```python
from build123d import *

# Parameters (mm, degrees)
EXTRUDE_1_DEPTH   = 2
HOLE_WIZARD_M61_D = 6.6
CHAMFER_1_SIZE    = 2


with BuildPart() as part:
    # Эскиз1 → Бобышка-Вытянуть1 (new body)
    with BuildSketch(Plane(origin=(0, 0, 0), x_dir=(1, 0, 0), z_dir=(0, 0, -1))):
        Polygon((0, 0), (0, 90), (90, 90), (90, 70), (20, 0), align=None)
    extrude(amount=EXTRUDE_1_DEPTH)

    # Отверстие с зазором M61 (through all)
    with Locations(Plane(origin=(0, 0, -2), x_dir=(1, 0, 0), z_dir=(0, 0, -1))):
        with Locations((40, 80), (10, 80), (10, 50), (10, 20), (70, 80), (40, 50)):
            Hole(HOLE_WIZARD_M61_D / 2)

    # Фаска1
    chamfer_1_edges = [part.edges().sort_by_distance(p)[0] for p in [
        (0, 0, -1),
        (0, -90, -1),
        (90, -90, -1),
    ]]
    chamfer(chamfer_1_edges, length=CHAMFER_1_SIZE)


solid = part.part
```
Input: part model. Units: mm. Frame: model coordinates. Coordinates: 2 decimals unless noted, no trailing zeros. Loops run counter-clockwise (first coordinate to the right, second up) from the corner with the lowest first, then second, coordinate; pieces in that order, holes last.
Q1. Mould query, pull axis Y, two halves, no side actions, for faces 1 (the flat face through (1, -1, -1)), 2 (the flat face through (36, -56, 0)), 3 (the cylindrical face through (12.619, -17.992, -0.986)), 4 (the flat face through (89, -89, -1)). Classes: +Y half, -Y half, draft (parallel to the pull), parting line (faces both ways), or undercut.
Results are:
face 1: +Y half
face 2: draft
face 3: undercut
face 4: -Y half
Q2. Line query: line 1 along Y through (x, z) = (10, -1.25); line 2 along X through (y, z) = (-80, -1.45); line 3 along Y through (x, z) = (38, -1.8). Output: solid intervals per line, ascending.
Results are:
line 1: y = -90 to -83.3, -76.7 to -53.3, -46.7 to -23.3, -16.7 to 0
line 2: x = 0 to 6.7, 13.3 to 36.7, 43.3 to 66.7, 73.3 to 90
line 3: y = -90 to -82.62, -77.38 to -52.62, -47.38 to -18
Q3. Section C-C, the plane z = -1.05. Return the cut outline in (x, y), and give its area (3 significant figures).
Results are:
outline: (0, -88) - (2, -90) - (88, -90) - (90, -88) - (90, -70) - (20, 0) - (2, 0) - (0, -2) - close; hole circle Ø6.6 at (10, -80); hole circle Ø6.6 at (10, -50); hole circle Ø6.6 at (10, -20); hole circle Ø6.6 at (40, -80); hole circle Ø6.6 at (40, -50); hole circle Ø6.6 at (70, -80)
area: 5,440 mm2
Q4. Section B-B, the plane y = -80. Return the cut outline in (x, z).
Results are:
outline: (0, -2) - (6.7, -2) - (6.7, 0) - (0, 0) - close; (13.3, -2) - (36.7, -2) - (36.7, 0) - (13.3, 0) - close; (43.3, -2) - (66.7, -2) - (66.7, 0) - (43.3, 0) - close; (73.3, -2) - (90, -2) - (90, 0) - (73.3, 0) - close
Q5. Section D-D, the plane x = 10. Return the cut outline in (y, z), and give its area (3 significant figures).
Results are:
outline: (-90, -2) - (-83.3, -2) - (-83.3, 0) - (-90, 0) - close; (-76.7, -2) - (-53.3, -2) - (-53.3, 0) - (-76.7, 0) - close; (-46.7, -2) - (-23.3, -2) - (-23.3, 0) - (-46.7, 0) - close; (-16.7, -2) - (0, -2) - (0, 0) - (-16.7, 0) - close
area: 140 mm2
Q6. Contact query for flat-ended pins moving along their axis: pin 1 (10.5 mm diameter, centred on x = 70, y = -80, fed in from -Z); pin 2 (4 mm diameter, centred on x = 10, y = -20, fed in from -Z). Output: stop coordinate, or through.
Results are:
pin 1: stops at z = -2
pin 2: passes through
Q7. Section A-A, the plane x = 40. Return the cut outline in (y, z), and give its area (3 significant figures).
Results are:
outline: (-90, -2) - (-83.3, -2) - (-83.3, 0) - (-90, 0) - close; (-76.7, -2) - (-53.3, -2) - (-53.3, 0) - (-76.7, 0) - close; (-46.7, -2) - (-20, -2) - (-20, 0) - (-46.7, 0) - close
area: 114 mm2
